CAD build for the part. Positions are in the model's coordinates, mm. A direction names the side the tool comes from. Coordinates: 2 decimals unless noted, no trailing zeros. Loops run counter-clockwise (first coordinate to the right, second up) from the corner with the lowest first, then second, coordinate; pieces in that order, holes last. Notation, with made-up numbers: (87.5, 18) -> (96.5, 18) arc R22 cw to (96.5, 30) -> close; hole circle Ø4 at (46, -1). An arc over 180 degrees is marked (long way). Answer as CSV lines item,"result". Start each with the question number.
from build123d import *

# Parameters (mm, degrees)
SKETCH_1_W          = 79
SKETCH_1_H          = 48
SKETCH_1_W_2        = 2.54
SKETCH_1_H_2        = 20.32
SKETCH_1_W_3        = 20
SKETCH_1_H_3        = 15
EXTRUDE_1_DEPTH     = 4
SKETCH_3_W          = 8
SKETCH_3_H          = 4
EXTRUDE_2_DEPTH     = 8
FILLET_1_R          = 2
SKETCH_5_R          = 3
CUT_EXTRUDE_1_DEPTH = 24
SKETCH2_W           = 8
SKETCH2_H           = 4
BOSS_EXTRUDE1_DEPTH = 8
FILLET1_R           = 2
CUT_EXTRUDE2_START  = -24
SKETCH3_R           = 3
CUT_EXTRUDE2_DEPTH  = 24
CHAMFER1_SIZE       = 3
CUT_EXTRUDE5_REACH  = 75.437
SKETCH8_R           = 1.55
BOSS_EXTRUDE4_DEPTH = 6
SKETCH10_W          = 17.5
SKETCH10_H          = 18
CUT_EXTRUDE6_DEPTH  = 1.5
BOSS_EXTRUDE5_DEPTH = 7


with BuildPart() as part:
    # Эскиз1 → Бобышка-Вытянуть1 (new body)
    with BuildSketch(Plane(origin=(0, 0, 0), x_dir=(1, 0, 0), z_dir=(0, 1, 0))):
        with Locations((39.5, 24)):
            Rectangle(SKETCH_1_W, SKETCH_1_H)
        with Locations((28.07, 12.66)):
            Rectangle(SKETCH_1_W_2, SKETCH_1_H_2, mode=Mode.SUBTRACT)
        with Locations((50.93, 12.66)):
            Rectangle(SKETCH_1_W_2, SKETCH_1_H_2, mode=Mode.SUBTRACT)
        with Locations((39.5, 37.5)):
            Rectangle(SKETCH_1_W_3, SKETCH_1_H_3, mode=Mode.SUBTRACT)
    extrude(amount=EXTRUDE_1_DEPTH)

    # Эскиз3 → Бобышка-Вытянуть2 (add)
    with BuildSketch(Plane(origin=(29.5, 0, 0), x_dir=(0, 0, -1), z_dir=(1, 0, 0))):
        with Locations((37.5, 6)):
            Rectangle(SKETCH_3_W, SKETCH_3_H)
    extrude(amount=-EXTRUDE_2_DEPTH)

    # Скругление1
    fillet_1_edges = [part.edges().sort_by_distance(p)[0] for p in [
        (25.5, 4, -41.5),
        (25.5, 4, -33.5),
    ]]
    fillet(fillet_1_edges, radius=FILLET_1_R)
    fillet_1_2_edges = [part.edges().sort_by_distance(p)[0] for p in [
        (25.5, 8, -41.5),
        (25.5, 8, -33.5),
    ]]
    fillet(fillet_1_2_edges, radius=FILLET_1_R - 0.0001)  # a hair under: the kernel refuses the full size

    # Эскиз5 → Вырез-Вытянуть1 (cut)
    with BuildSketch(Plane.ZY):
        with Locations((-37.5, 4)):
            Circle(SKETCH_5_R)
    extrude(amount=-CUT_EXTRUDE_1_DEPTH, mode=Mode.SUBTRACT)

    # Sketch2 → Boss-Extrude1 (add)
    with BuildSketch(Plane.ZY.offset(-49.5)):
        with Locations((-37.5, 6)):
            Rectangle(SKETCH2_W, SKETCH2_H)
    extrude(amount=-BOSS_EXTRUDE1_DEPTH)

    # Fillet1
    fillet1_edges = [part.edges().sort_by_distance(p)[0] for p in [
        (53.5, 4, -33.5),
    ]]
    fillet(fillet1_edges, radius=FILLET1_R)
    fillet1_2_edges = [part.edges().sort_by_distance(p)[0] for p in [
        (53.5, 4, -41.5),
    ]]
    fillet(fillet1_2_edges, radius=FILLET1_R)
    fillet1_3_edges = [part.edges().sort_by_distance(p)[0] for p in [
        (53.5, 8, -33.5),
    ]]
    fillet(fillet1_3_edges, radius=FILLET1_R - 0.0001)  # a hair under: the kernel refuses the full size
    fillet1_4_edges = [part.edges().sort_by_distance(p)[0] for p in [
        (53.5, 8, -41.5),
    ]]
    fillet(fillet1_4_edges, radius=FILLET1_R - 0.0001)  # a hair under: the kernel refuses the full size

    # Sketch3 → Cut-Extrude2 (cut)
    with BuildSketch(Plane(origin=(79, 0, 0), x_dir=(0, 0, -1), z_dir=(1, 0, 0)).offset(CUT_EXTRUDE2_START)):
        with Locations(Location((37.5, 4, 0), (0, 0, 180))):
            Circle(SKETCH3_R)
    extrude(amount=CUT_EXTRUDE2_DEPTH, mode=Mode.SUBTRACT)

    # Chamfer1
    chamfer1_edges = [part.edges().sort_by_distance(p)[0] for p in [
        (39.5, 4, -30),
        (39.5, 4, -45),
    ]]
    chamfer(chamfer1_edges, length=CHAMFER1_SIZE - 0.0001)  # a hair under: the kernel refuses the full size

    # Cut-Extrude5: up to this face of the body (flat: up to its plane)
    cut_extrude5_end = Plane(part.part.faces().sort_by_distance((24, 4, -37.5))[0])
    # Sketch8 → Cut-Extrude5 (cut, up to the picked face)
    with BuildSketch(Plane(origin=(55, 0, 0), x_dir=(0, 0, -1), z_dir=(1, 0, 0)), mode=Mode.PRIVATE) as cut_extrude5_sk1:
        with Locations((37.5, 4)):
            Circle(SKETCH8_R)
    cut_extrude5_tool1 = split(extrude(cut_extrude5_sk1.sketch, amount=-CUT_EXTRUDE5_REACH, mode=Mode.PRIVATE), bisect_by=cut_extrude5_end, keep=Keep.BOTH, mode=Mode.PRIVATE)
    add(cut_extrude5_tool1.solids().sort_by(Axis((55, 4, -37.5), (-1, 0, 0)))[0], mode=Mode.SUBTRACT)

    # Sketch9 → Boss-Extrude4 (add)
    with BuildSketch(Plane(origin=(0, 0, -48), x_dir=(-1, 0, 0), z_dir=(0, 0, -1))):
        with BuildLine():
            Line((-79, 0), (-63, 0))
            Line((-63, 0), (-63, -7.5))
            ThreePointArc((-63, -7.5), (-63.129574487, -8.934016124), (-63.514100561, -10.321579273))
            Line((-63.514100561, -10.321579273), (-65.385575421, -9.616184455))
            ThreePointArc((-65.385575421, -9.616184455), (-71, -1.5), (-76.614424579, -9.616184455))
            Line((-76.614424579, -9.616184455), (-78.485899439, -10.321579273))
            ThreePointArc((-78.485899439, -10.321579273), (-78.870425513, -8.934016124), (-79, -7.5))
            Line((-79, -7.5), (-79, 0))
        make_face()
        with BuildLine():
            Line((-13.614424579, -9.616184455), (-15.485899439, -10.321579273))
            ThreePointArc((-15.485899439, -10.321579273), (-15.870425513, -8.934016124), (-16, -7.5))
            Line((-16, -7.5), (-16, 0))
            Line((-16, 0), (0, 0))
            Line((0, 0), (0, -7.5))
            ThreePointArc((0, -7.5), (-0.129574487, -8.934016124), (-0.514100561, -10.321579273))
            Line((-0.514100561, -10.321579273), (-2.385575421, -9.616184455))
            ThreePointArc((-2.385575421, -9.616184455), (-8, -1.5), (-13.614424579, -9.616184455))
        make_face()
    extrude(amount=-BOSS_EXTRUDE4_DEPTH)

    # Sketch10 → Cut-Extrude6 (cut)
    with BuildSketch(Plane(origin=(0, 4, 0), x_dir=(1, 0, 0), z_dir=(0, 1, 0))):
        with Locations((39.5, 9)):
            Rectangle(SKETCH10_W, SKETCH10_H)
    extrude(amount=-CUT_EXTRUDE6_DEPTH, mode=Mode.SUBTRACT)

    # Sketch13 → Boss-Extrude5 (add)
    with BuildSketch(Plane.XY.offset(-10)):
        with BuildLine():
            Line((0, 0), (16, 0))
            Line((16, 0), (16, -7.5))
            ThreePointArc((16, -7.5), (15.870425513, -8.934016124), (15.485899439, -10.321579273))
            Line((15.485899439, -10.321579273), (13.614424579, -9.616184455))
            ThreePointArc((13.614424579, -9.616184455), (8, -1.5), (2.385575421, -9.616184455))
            Line((2.385575421, -9.616184455), (0.514100561, -10.321579273))
            ThreePointArc((0.514100561, -10.321579273), (0.129574487, -8.934016124), (0, -7.5))
            Line((0, -7.5), (0, 0))
        make_face()
        with BuildLine():
            Line((63, 0), (63, -7.5))
            ThreePointArc((63, -7.5), (63.129574487, -8.934016124), (63.514100561, -10.321579273))
            Line((63.514100561, -10.321579273), (65.385575421, -9.616184455))
            ThreePointArc((65.385575421, -9.616184455), (71, -1.5), (76.614424579, -9.616184455))
            Line((76.614424579, -9.616184455), (78.485899439, -10.321579273))
            ThreePointArc((78.485899439, -10.321579273), (78.870425513, -8.934016124), (79, -7.5))
            Line((79, -7.5), (79, 0))
            Line((79, 0), (63, 0))
        make_face()
    extrude(amount=BOSS_EXTRUDE5_DEPTH)


solid = part.part
Item 1: Saw through at D-D (z = -11.5). Write the cut outline in (x, y), plus the area to 3 significant figures.
Item 2: Flat gauge pins, fed straight in: pin 1 Ø3 at (x, z) = (22.5, -13.5) entering from +Y; pin 2 Ø5 at (y, z) = (4, -37.5) entering from +X; pin 3 Ø3 at (x, y) = (5, -5.5) entering from -Z; pin 4 Ø2 at (y, z) = (5.5, -39.5) entering from -X. Where does each tip first touch, or does it go through?
Item 3: Saw through at C-C (y = -4). Count the separate pieces of the cut face and the enclosed holes in it, plus the area to 3 significant figures.
Item 4: Saw through at A-A (z = -37.5). Write the cut outline in (x, y), plus the area to 3 significant figures.
Item 5: Wall check: probe 1 along X at (y, z) = (-7.5, -45.05); probe 2 along X at (y, z) = (3.25, -16); probe 3 along X at (y, z) = (3, -29). Give the ranges that are in metal, low to high.
Item 6: Which spindle directions (+Z, -Z, +X, -X, +Y, -Y) get a long thin tool onto all of the face, cutting with end or side? Do faces 1 (the face through (64.437, -9.974, -6.549)), 2 (the face through (39, 2, -29)), 3 (the face through (28, 2, -2.5)), 4 (the face through (9.9, -1.6, -10)). Say none if no direction does.
Item 7: Two-plate mould, pull along Z, no slides. Class faces 5 (the face through (29.5, 2, -37)), 6 (the face through (64.437, -9.974, -45.042)), 7 (the face through (53.56, 4.57, -42.1)), 8 (the face through (69.1, -1.6, -3)): pulls with the +Z half, pulls with the -Z half, needs draft (parallel to the pull), parting line crosses it, or undercut.
Geometry check:
1,outline,"(0, 0) -> (26.8, 0) -> (26.8, 4) -> (0, 4) -> close; (29.34, 0) -> (49.66, 0) -> (49.66, 4) -> (48.25, 4) -> (48.25, 2.5) -> (30.75, 2.5) -> (30.75, 4) -> (29.34, 4) -> close; (52.2, 0) -> (79, 0) -> (79, 4) -> (52.2, 4) -> close"
1,area,"269 mm2"
2,pin 1,"y = 4"
2,pin 2,"x = 55"
2,pin 3,"through"
2,pin 4,"x = 21.5"
3,separate pieces,"8"
3,enclosed holes,"0"
3,area,"163 mm2"
4,outline,"(0, 0) -> (29.5, 0) -> (29.5, 2.45) -> (24, 2.45) -> (24, 1) -> (0, 1) -> close; (21.5, 7) -> (24, 7) -> (24, 5.55) -> (29.5, 5.55) -> (29.5, 8) -> (21.5, 8) -> close; (49.5, 0) -> (79, 0) -> (79, 1) -> (55, 1) -> (55, 2.45) -> (49.5, 2.45) -> close; (49.5, 5.55) -> (55, 5.55) -> (55, 7) -> (57.5, 7) -> (57.5, 8) -> (49.5, 8) -> close"
4,area,"107 mm2"
5,probe 1,"0 to 2, 14 to 16, 63 to 65, 77 to 79"
5,probe 2,"0 to 26.8, 29.34 to 30.75, 48.25 to 49.66, 52.2 to 79"
5,probe 3,"0 to 29.5, 49.5 to 79"
6,face 1,"+Z, -Z, -Y"
6,face 2,"+Y"
6,face 3,"+Y, -Y"
6,face 4,"+X, -X, -Y"
7,face 5,"undercut"
7,face 6,"needs draft"
7,face 7,"pulls with the -Z half"
7,face 8,"pulls with the +Z half"
